from build123d import *

# Parameters (mm, degrees)
ESQUISSE1_R        = 156
ESQUISSE1_R_2      = 6.75
ESQUISSE1_W        = 40
ESQUISSE1_H        = 80
BOSS_EXTRU_1_DEPTH = 10


with BuildPart() as part:
    # Esquisse1 → Boss.-Extru.1 (new body)
    with BuildSketch(Plane(origin=(0, 0, 0), x_dir=(0, 0, -1), z_dir=(1, 0, 0))):
        Circle(ESQUISSE1_R)
        with Locations((127.441573184, -41.408277246)):
            Circle(ESQUISSE1_R_2, mode=Mode.SUBTRACT)
        with Locations((134, 0)):
            Circle(ESQUISSE1_R_2, mode=Mode.SUBTRACT)
        with Locations((108.408277246, -78.763223807)):
            Circle(ESQUISSE1_R_2, mode=Mode.SUBTRACT)
        with Locations((78.763223807, -108.408277246)):
            Circle(ESQUISSE1_R_2, mode=Mode.SUBTRACT)
        with Locations((41.408277246, -127.441573184)):
            Circle(ESQUISSE1_R_2, mode=Mode.SUBTRACT)
        with Locations((0, -134)):
            Circle(ESQUISSE1_R_2, mode=Mode.SUBTRACT)
        with Locations((-41.408277246, -127.441573184)):
            Circle(ESQUISSE1_R_2, mode=Mode.SUBTRACT)
        with Locations((-78.763223807, -108.408277246)):
            Circle(ESQUISSE1_R_2, mode=Mode.SUBTRACT)
        with Locations((-108.408277246, -78.763223807)):
            Circle(ESQUISSE1_R_2, mode=Mode.SUBTRACT)
        with Locations((-127.441573184, -41.408277246)):
            Circle(ESQUISSE1_R_2, mode=Mode.SUBTRACT)
        with Locations((-134, 0)):
            Circle(ESQUISSE1_R_2, mode=Mode.SUBTRACT)
        with Locations((-127.441573184, 41.408277246)):
            Circle(ESQUISSE1_R_2, mode=Mode.SUBTRACT)
        with Locations((-108.408277246, 78.763223807)):
            Circle(ESQUISSE1_R_2, mode=Mode.SUBTRACT)
        with Locations((-78.763223807, 108.408277246)):
            Circle(ESQUISSE1_R_2, mode=Mode.SUBTRACT)
        with Locations((-41.408277246, 127.441573184)):
            Circle(ESQUISSE1_R_2, mode=Mode.SUBTRACT)
        with Locations((0, 134)):
            Circle(ESQUISSE1_R_2, mode=Mode.SUBTRACT)
        with Locations((41.408277246, 127.441573184)):
            Circle(ESQUISSE1_R_2, mode=Mode.SUBTRACT)
        with Locations((78.763223807, 108.408277246)):
            Circle(ESQUISSE1_R_2, mode=Mode.SUBTRACT)
        with Locations((108.408277246, 78.763223807)):
            Circle(ESQUISSE1_R_2, mode=Mode.SUBTRACT)
        with Locations((127.441573184, 41.408277246)):
            Circle(ESQUISSE1_R_2, mode=Mode.SUBTRACT)
        with Locations((-80, 0)):
            Rectangle(ESQUISSE1_W, ESQUISSE1_H, mode=Mode.SUBTRACT)
        with Locations((80, 0)):
            Rectangle(ESQUISSE1_W, ESQUISSE1_H, mode=Mode.SUBTRACT)
    extrude(amount=BOSS_EXTRU_1_DEPTH)


solid = part.part
Source: CAD feature listing. Evaluate the final solid. Frame: model axes, mm. A direction names the side the tool comes from. Coordinates: 2 decimals unless noted, no trailing zeros. Loops run counter-clockwise (first coordinate to the right, second up) from the corner with the lowest first, then second, coordinate; pieces in that order, holes last. Notation, with made-up numbers: M 10.5,41 L 68.5,41 A16 cw 68.5,53 Z; hole C 24,28 d10. An arc over 180 degrees is marked long. Answer in a Markdown table with one row per item.
Q1. Section D-D on y = -56.5. Return the cut outline in (x, z).
Answers below:
| item | result |
|---|---|
| outline | M 0,-145.41 L 10,-145.41 L 10,145.41 L 0,145.41 Z |
Q2. First-contact query: pin 1 (5 mm diameter, centred on x = 4, z = -89.5, fed in from -Y); pin 2 (2 mm diameter, centred on y = 13, z = 19.5, fed in from -X); pin 3 (2 mm diameter, centred on x = 5, z = 107.5, fed in from +Y); pin 4 (5 mm diameter, centred on x = 7, y = 64, fed in from +Z). Flat tips, straight axial feed; report the tip coordinate or a pass-through.
Answers below:
| item | result |
|---|---|
| pin 1 | stops at y = -129.49 |
| pin 2 | stops at x = 0 |
| pin 3 | stops at y = 113.99 |
| pin 4 | stops at z = 143.37 |
Q3. Set-up query: faces 4 (the flat face through (10, 2, 2)), 5 (the flat face through (5, -40, 80)). Return all of +Z, -Z, +X, -X, +Y, -Y with unobstructed straight access to the full face (end or side cutting, diameter ignored); none if empty.
Answers below:
| item | result |
|---|---|
| face 4 | +Z, -Z, +X, +Y, -Y |
| face 5 | +X, -X |
Q4. Section B-B on z = -95.5. Return the cut outline in (x, y).
Answers below:
| item | result |
|---|---|
| outline | M 0,-123.35 L 10,-123.35 L 10,-40 L 0,-40 Z; M 0,40 L 10,40 L 10,123.35 L 0,123.35 Z |
Q5. Section C-C on x = 6.25. State how many separate pieces and enclosed holes the cut face has, plus the area to 3 significant figures.
Answers below:
| item | result |
|---|---|
| separate pieces | 1 |
| enclosed holes | 22 |
| area | 67,200 mm^2 |
Q6. Section A-A on z = 0. Return the cut outline in (x, y), plus the area to 3 significant figures.
Answers below:
| item | result |
|---|---|
| outline | M 0,-156 L 10,-156 L 10,-140.75 L 0,-140.75 Z; M 0,-127.25 L 10,-127.25 L 10,127.25 L 0,127.25 Z; M 0,140.75 L 10,140.75 L 10,156 L 0,156 Z |
| area | 2,850 mm^2 |
Q7. Draft query along Y for faces 1 (the cylindrical face through (4.93, 102.42, -81.88)), 2 (the cylindrical face through (4.93, 154.672, 20.308)), 3 (the flat face through (0, 2, 2)). Return one class per face: pulls with the +Y half, pulls with the -Y half, needs draft (parallel to the pull), parting line crosses it, or undercut.
Answers below:
| item | result |
|---|---|
| face 1 | undercut |
| face 2 | parting line crosses it |
| face 3 | needs draft |
Q8. Ray query, probe 1 along Y at (x, z) = (4.25, 0); probe 2 along Z at (x, y) = (2.5, -41.5); probe 3 along Y at (x, z) = (3, 104.5). Return the intervals inside material, ascending. Write a range as from..to.
Answers below:
| item | result |
|---|---|
| probe 1 | y = -156..-140.75, -127.25..127.25, 140.75..156 |
| probe 2 | z = -150.38..-134.19, -120.69..120.69, 134.19..150.38 |
| probe 3 | y = -115.83..-84.27, -73.26..73.26, 84.27..115.83 |
